The listing builds one solid part. Answer for the finished solid, in the listing's coordinates (mm). A direction names the side the tool comes from. Coordinates: 2 decimals unless noted, no trailing zeros. Order: outer loops, then holes, each group sorted by start corner. A loop starts at its lowest first (then second) coordinate and runs counter-clockwise, first axis right, second up. Notation, with made-up numbers: (-5, 85) -> (12, 85) arc R6 cw to (12, 96) -> close; hole circle Ø3 at (31.5, 3.5). An arc over 180 degrees is marked (long way). Answer in a Markdown table with one row per item.
```python
from build123d import *

# Parameters (mm, degrees)
SKETCH1_W           = 12.5
SKETCH1_H           = 10
SKETCH1_W_2         = 30
SKETCH1_H_2         = 200
SKETCH1_W_3         = 10
BOSS_EXTRUDE1_DEPTH = 5


with BuildPart() as part:
    # Sketch1 → Boss-Extrude1 (new body)
    with BuildSketch(Plane(origin=(0, 0, 0), x_dir=(1, 0, 0), z_dir=(0, 1, 0))):
        with Locations((83.16678375, -31.56250034)):
            Rectangle(SKETCH1_W, SKETCH1_H)
        with Locations((83.16678375, 68.43749966)):
            Rectangle(SKETCH1_W_2, SKETCH1_H_2)
        with Locations((83.16678375, 168.43749966)):
            Rectangle(SKETCH1_W_3, SKETCH1_H)
    extrude(amount=BOSS_EXTRUDE1_DEPTH)


solid = part.part
```
(1) Find the intervals of material crossed by line 1 along Z through (x, y) = (72.25, 4.75); line 2 along Z through (x, y) = (88.5, 4.6), in increasing order. Write a range as from..to.
Check values:
| item | result |
|---|---|
| line 1 | -168.44..31.56 |
| line 2 | -168.44..36.56 |
(2) Flat-ended cylindrical pins translate along their axes: pin 1 (1.5 mm diameter, centred on x = 71, y = 3.5, fed in from +Z); pin 2 (12 mm diameter, centred on x = 93, z = -141, fed in from -Y); pin 3 (2.5 mm diameter, centred on x = 91.5, y = 2.5, fed in from -Z); pin 4 (2.5 mm diameter, centred on y = 3, z = 35.5, fed in from +X). Find the tip coordinate at first contact, or state that the pin passes through.
Check values:
| item | result |
|---|---|
| pin 1 | z = 31.56 |
| pin 2 | y = 0 |
| pin 3 | z = -168.44 |
| pin 4 | x = 89.42 |
(3) A cutting plane is placed at A-A, the plane y = 1.55. Determine the outline of the cut face in (x, z), then the cut area to 3 significant figures.
Check values:
| item | result |
|---|---|
| outline | (68.17, -168.44) -> (78.17, -168.44) -> (78.17, -173.44) -> (88.17, -173.44) -> (88.17, -168.44) -> (98.17, -168.44) -> (98.17, 31.56) -> (89.42, 31.56) -> (89.42, 36.56) -> (76.92, 36.56) -> (76.92, 31.56) -> (68.17, 31.56) -> close |
| area | 6,110 mm² |
(4) A cutting plane is placed at B-B, the plane x = 72.5. Determine the outline of the cut face in (y, z), then the cut area to 3 significant figures.
Check values:
| item | result |
|---|---|
| outline | (0, -168.44) -> (5, -168.44) -> (5, 31.56) -> (0, 31.56) -> close |
| area | 1,000 mm² |
(5) Which of the six approach directions +Z, -Z, +X, -X, +Y, -Y give full straight-line access (tool end or side, diameter ignored) to faces 1 (the flat face through (73, 2, -168.437)), 2 (the flat face through (93, 2, -168.437)), 3 (the flat face through (72, 2, 31.563)), 4 (the flat face through (94, 2, 31.563))?
Check values:
| item | result |
|---|---|
| face 1 | -Z, -X, +Y, -Y |
| face 2 | -Z, +X, +Y, -Y |
| face 3 | +Z, -X, +Y, -Y |
| face 4 | +Z, +X, +Y, -Y |
